Can you work these out from the model? Positions are in its coordinate system, mm. Round coordinates to 2 decimals unless told otherwise and drop trailing zeros. Write each loop counter-clockwise with the first axis right and the second up, starting at its lowest first coordinate (ties: lowest second). Pieces come first, ordered by that corner, then holes. Notation, with made-up numbers: (55.5, 16) -> (103.5, 16) arc R8 ccw to (103.5, 28) -> close; hole circle Ø11 at (4.25, -12.5). An arc over 180 degrees is marked (long way). Use CSV: the item, a comma, the result in double quotes.
```python
from build123d import *

# Parameters (mm, degrees)
SKETCH2_W                = 110
SKETCH2_H                = 55
BOSS_EXTRUDE1_DEPTH      = 1.5875
M4_CLEARANCE_HOLE1_D     = 4.5
M4_CLEARANCE_HOLE2_D     = 4.5
M4_CLEARANCE_HOLE2_DEPTH = 10.1
M4_CLEARANCE_HOLE2_TIP   = 1.351936393
M4_CLEARANCE_HOLE3_D     = 4.5
CHAMFER1_SIZE            = 15
FILLET1_R                = 15
SKETCH9_R                = 4
CUT_EXTRUDE1_DEPTH       = 4.175
M5X0_8_TAPPED_HOLE1_D    = 4.2


with BuildPart() as part:
    # Sketch2 → Boss-Extrude1 (new body, symmetric)
    with BuildSketch(Plane(origin=(0, 0, 0), x_dir=(1, 0, 0), z_dir=(0, 1, 0))):
        Rectangle(SKETCH2_W, SKETCH2_H)
    extrude(amount=BOSS_EXTRUDE1_DEPTH, both=True)

    # M4 Clearance Hole1 (through all)
    with Locations(Plane(origin=(0, 1.5875, 0), x_dir=(1, 0, 0), z_dir=(0, 1, 0))):
        with Locations((-37.5, -17), (37.5, -17)):
            Hole(M4_CLEARANCE_HOLE1_D / 2)

    # M4 Clearance Hole2
    with Locations(Plane(origin=(0, 1.5875, 0), x_dir=(1, 0, 0), z_dir=(0, 1, 0))):
        with Locations((0, 22.5)):
            Hole(M4_CLEARANCE_HOLE2_D / 2, depth=M4_CLEARANCE_HOLE2_DEPTH)
            with Locations((0, 0, -(M4_CLEARANCE_HOLE2_DEPTH + M4_CLEARANCE_HOLE2_TIP / 2))):  # 118° drill point
                Cone(0, M4_CLEARANCE_HOLE2_D / 2, M4_CLEARANCE_HOLE2_TIP, mode=Mode.SUBTRACT)

    # M4 Clearance Hole3 (through all)
    with Locations(Plane(origin=(0, 1.5875, 0), x_dir=(1, 0, 0), z_dir=(0, 1, 0))):
        with Locations((-46, 5.5), (46, 5.5), (21, 20.5), (-21, 20.5)):
            Hole(M4_CLEARANCE_HOLE3_D / 2)

    # Chamfer1
    chamfer1_edges = [part.edges().sort_by_distance(p)[0] for p in [
        (-55, 0, -27.5),
        (55, 0, -27.5),
    ]]
    chamfer(chamfer1_edges, length=CHAMFER1_SIZE)

    # Fillet1
    fillet1_edges = [part.edges().sort_by_distance(p)[0] for p in [
        (-55, 0, -12.5),
        (40, 0, -27.5),
        (-40, 0, -27.5),
        (55, 0, -12.5),
        (55, 0, 27.5),
        (-55, 0, 27.5),
    ]]
    fillet(fillet1_edges, radius=FILLET1_R)

    # Sketch9 → Cut-Extrude1 (cut, through all)
    with BuildSketch(Plane(origin=(0, 1.5875, 0), x_dir=(1, 0, 0), z_dir=(0, 1, 0))):
        with Locations((-16, -5.635528726)):
            Circle(SKETCH9_R)
    extrude(amount=-CUT_EXTRUDE1_DEPTH, mode=Mode.SUBTRACT)

    # M5x0.8 Tapped Hole1 (through all)
    with Locations(Plane(origin=(0, 1.5875, 0), x_dir=(1, 0, 0), z_dir=(0, 1, 0))):
        with Locations((16, -5.635528726)):
            Hole(M5X0_8_TAPPED_HOLE1_D / 2)


solid = part.part
```
Q1. Suppose I cut it at C-C (z = 17). Write out the boundary of the cut face in (x, y), and give its area (3 significant figures).
Resolved:
outline,"(-54.31, -1.59) -> (-39.75, -1.59) -> (-39.75, 1.59) -> (-54.31, 1.59) -> close; (-35.25, -1.59) -> (35.25, -1.59) -> (35.25, 1.59) -> (-35.25, 1.59) -> close; (39.75, -1.59) -> (54.31, -1.59) -> (54.31, 1.59) -> (39.75, 1.59) -> close"
area,"316 mm^2"
Q2. Suppose I cut it at B-B (y = -0.35). Count the separate pieces of the cut face and the enclosed holes in it, and give its area (3 significant figures).
Resolved:
separate pieces,"1"
enclosed holes,"9"
area,"5,530 mm^2"
Q3. Suppose I cut it at A-A (x = -16). Write out the boundary of the cut face in (y, z), and give its area (3 significant figures).
Resolved:
outline,"(-1.59, -27.5) -> (1.59, -27.5) -> (1.59, 1.64) -> (-1.59, 1.64) -> close; (-1.59, 9.64) -> (1.59, 9.64) -> (1.59, 27.5) -> (-1.59, 27.5) -> close"
area,"149 mm^2"
Q4. Suppose I cut it at D-D (x = 46). Write out the boundary of the cut face in (y, z), and give its area (3 significant figures).
Resolved:
outline,"(-1.59, -21.5) -> (1.59, -21.5) -> (1.59, -7.75) -> (-1.59, -7.75) -> close; (-1.59, -3.25) -> (1.59, -3.25) -> (1.59, 26.25) -> (-1.59, 26.25) -> close"
area,"137 mm^2"
Q5. Please list where these lines run through material, in increasing order: probe 1 along Z at (x, y) = (-16, 0.15); probe 2 along X at (y, z) = (0.6, -7.5); probe 3 along X at (y, z) = (-0.9, -21).
Resolved:
probe 1,"z = -27.5 to 1.64, 9.64 to 27.5"
probe 2,"x = -54.95 to -47.03, -44.97 to 44.97, 47.03 to 54.95"
probe 3,"x = -46.5 to -23.19, -18.81 to -1.68, 1.68 to 18.81, 23.19 to 46.5"
Q6. If we mould it in two halves opening along Z, with no side actions, what happens to faces 1 (the face through (-39.603, -0.022, -26.326)), 2 (the face through (-1, 1.588, 0)), 3 (the face through (19.962, -0.022, -18.504)), 4 (the face through (50.49, 0.02, 23.22))? For each: released by +Z, released by -Z, zero draft, split by the parting line, or undercut.
Resolved:
face 1,"released by -Z"
face 2,"zero draft"
face 3,"undercut"
face 4,"released by +Z"
